Can you work these out from the model? Positions are in its coordinate system, mm. Face numbers are marked on the shaded views. Coordinates: 2 decimals unless noted, no trailing zeros. Order: outer loops, then holes, each group sorted by start corner. A loop starts at its lowest first (then second) coordinate and runs counter-clockwise, first axis right, second up. Notation, with made-up numbers: M 0,-14.75 L 49,-14.75 A12 cw 49,-1.75 Z; hole C 34,67.25 d4. An arc over 180 degrees is marked long. Answer as a JSON object with one key per item and string values.
from build123d import *

# Parameters (mm, degrees)
SKETCH1_W           = 60
SKETCH1_H           = 34
BOSS_EXTRUDE1_DEPTH = 16
BOSS_EXTRUDE2_DEPTH = 40
CUT_EXTRUDE2_DEPTH  = 40
SKETCH2_R           = 5
CUT_EXTRUDE1_DEPTH  = 72.274118725
FILLET1_R           = 6
CUT_EXTRUDE3_DEPTH  = 72.274118798


with BuildPart() as part:
    # Sketch1 → Boss-Extrude1 (new body)
    with BuildSketch(Plane(origin=(0, 0, 0), x_dir=(1, 0, 0), z_dir=(0, 1, 0))):
        with Locations((30, 17)):
            Rectangle(SKETCH1_W, SKETCH1_H)
    extrude(amount=BOSS_EXTRUDE1_DEPTH)

    # Sketch3 → Boss-Extrude2 (add)
    with BuildSketch(Plane.ZY):
        with BuildLine():
            Line((-34, 16), (-32, 18))
            ThreePointArc((-32, 18), (-30.88035776, 16.958314663), (-29.68857754, 16))
            Line((-29.68857754, 16), (-34, 16))
        make_face()
        with BuildLine():
            Line((-2, 18), (0, 16))
            Line((0, 16), (-4.31142246, 16))
            ThreePointArc((-4.31142246, 16), (-3.11964224, 16.958314663), (-2, 18))
        make_face()
    extrude(amount=-BOSS_EXTRUDE2_DEPTH)

    # Sketch4 → Cut-Extrude2 (cut)
    with BuildSketch(Plane.ZY):
        with BuildLine():
            Line((-19.472144861, 33), (-38.213203436, 33))
            ThreePointArc((-38.213203436, 33), (-17, 11.786796564), (4.213203436, 33))
            Line((4.213203436, 33), (-19.472144861, 33))
        make_face()
    extrude(amount=-CUT_EXTRUDE2_DEPTH, mode=Mode.SUBTRACT)

    # Sketch2 → Cut-Extrude1 (cut, through all)
    with BuildSketch(Plane.XY):
        with Locations((46, 16)):
            Circle(SKETCH2_R)
    extrude(amount=-CUT_EXTRUDE1_DEPTH, mode=Mode.SUBTRACT)

    # Fillet1
    fillet1_edges = [part.edges().sort_by_distance(p)[0] for p in [
        (0, 8, -34),
        (60, 8, -34),
        (60, 8, 0),
        (0, 8, 0),
    ]]
    fillet(fillet1_edges, radius=FILLET1_R)

    # Sketch5 → Cut-Extrude3 (cut, through all)
    with BuildSketch(Plane.XY):
        Polygon((50.705913613, 14.310509822), (60, 12.692705636), (60, 16), (51, 16), align=None)
    extrude(amount=-CUT_EXTRUDE3_DEPTH, mode=Mode.SUBTRACT)


solid = part.part
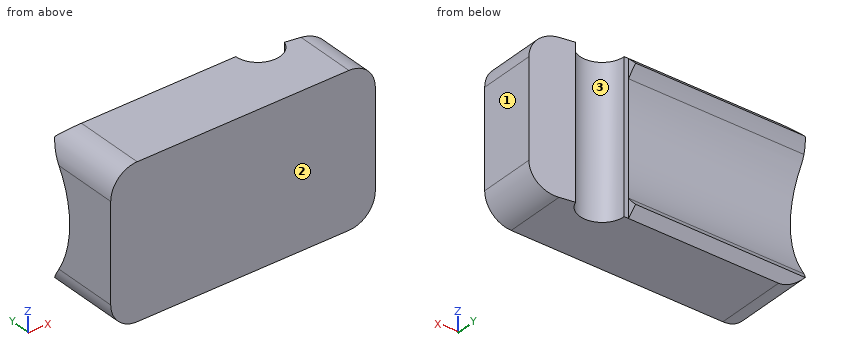
Item 1: I'm going to push flat-ended pins straight in: pin 1 (1 mm diameter, centred on x = 20.5, z = -4.5, fed in from +Y); pin 2 (1.1 mm diameter, centred on x = 40.5, z = -14.5, fed in from +Y); pin 3 (3.5 mm diameter, centred on y = 15, z = -14.5, fed in from -X). Where does each tip first touch, or does it pass through?
Answers follow:
{"pin 1": "stops at y = 16.24", "pin 2": "stops at y = 16", "pin 3": "stops at x = 40"}
Item 2: Please list where these lines run through material, in increasing order: line 1 (Y direction, x = 20, z = -28); line 2 (Y direction, x = 3.5, z = -17); line 3 (X direction, y = 11.75, z = -4).
Answers follow:
{"line 1": "y = 0 to 14.86", "line 2": "y = 0 to 11.79", "line 3": "x = 0.34 to 43.37, 48.63 to 59.66"}
Item 3: If we mould it in two halves opening along X, with no side actions, what happens to the marked faces 1, 2 and 3? For each: pulls with the +X half, pulls with the -X half, needs draft (parallel to the pull), parting line crosses it, or undercut.
Answers follow:
{"face 1": "pulls with the +X half", "face 2": "needs draft", "face 3": "undercut"}
Item 4: I want a section at A-A, the plane x = 34.5. Write out the boundary of the cut face in (y, z).
Answers follow:
{"outline": "M 0,-34 L 16,-34 L 18,-32 A21.21 cw 18,-2 L 16,0 L 0,0 Z"}
Item 5: I want a section at B-B, the plane y = 8. Write out the boundary of the cut face in (x, z).
Answers follow:
{"outline": "M 0,-28 A6 ccw 6,-34 L 54,-34 A6 ccw 60,-28 L 60,-6 A6 ccw 54,0 L 6,0 A6 ccw 0,-6 Z"}
